Drawing for the job (mm, zero at the part's lowest x, y, z). A direction names the side the tool comes from. Coordinates: 2 decimals unless noted, no trailing zeros. Write each loop counter-clockwise with the first axis right and the second up, starting at its lowest first coordinate (ties: lowest second). Pieces come first, ordered by that corner, then holes. Notation, with made-up numbers: (20, -33) -> (57, -33) arc R28 ccw to (57, -13) -> close; hole circle Ø7 at (22.5, 56). An arc over 180 degrees is marked (long way). Answer as CSV lines item,"result".
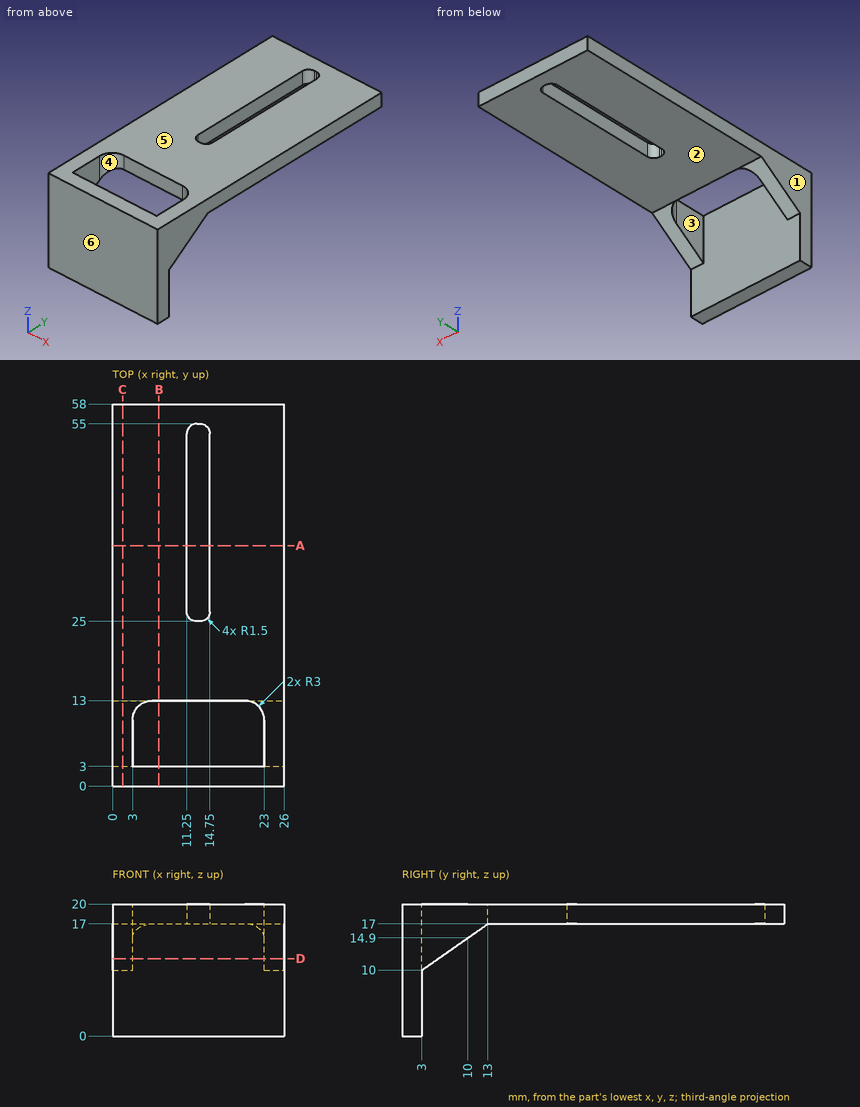
Item 1: 3-axis set-ups, long thin cutter, end or side, ignore diameter. For the marked faces 1, 2 and 3: which of +Z, -Z, +X, -X, +Y, -Y reach the whole face in a straight line?
Answer below:
face 1,"+Z, -Z, -X, +Y, -Y"
face 2,"-Z, +X, -X, +Y"
face 3,"+Z, -Z"
Item 2: Saw through at B-B on x = 7. Give the cut face in (y, z), and give its area (3 significant figures).
Answer below:
outline,"(0, 0) -> (3, 0) -> (3, 20) -> (0, 20) -> close; (13, 17) -> (58, 17) -> (58, 20) -> (13, 20) -> close"
area,"195 mm2"
Item 3: Saw through at C-C on x = 1.5. Give the cut face in (y, z).
Answer below:
outline,"(0, 0) -> (3, 0) -> (3, 10) -> (13, 17) -> (58, 17) -> (58, 20) -> (0, 20) -> close"
Item 4: Wall check: line 1 (Y direction, x = 12.75, z = 18.5); line 2 (X direction, y = 48.5, z = 19.25); line 3 (Y direction, x = 7, z = 18.75). Give the ranges that are in metal, low to high. Write a range as from..to.
Answer below:
line 1,"y = 0..3, 13..25, 55..58"
line 2,"x = 0..11.25, 14.75..26"
line 3,"y = 0..3, 13..58"
Item 5: Saw through at D-D on z = 11.75. Give the cut face in (x, y).
Answer below:
outline,"(0, 0) -> (26, 0) -> (26, 5.5) -> (23, 5.5) -> (23, 3) -> (3, 3) -> (3, 5.5) -> (0, 5.5) -> close"
Item 6: Saw through at A-A on y = 36.5. Give the cut face in (x, z), and give its area (3 significant figures).
Answer below:
outline,"(0, 17) -> (11.25, 17) -> (11.25, 20) -> (0, 20) -> close; (14.75, 17) -> (26, 17) -> (26, 20) -> (14.75, 20) -> close"
area,"67.5 mm2"
Item 7: Two-plate mould, pull along Y, no slides. Class the marked faces 4, 5 and 6: pulls with the +Y half, pulls with the -Y half, needs draft (parallel to the pull), parting line crosses it, or undercut.
Answer below:
face 4,"undercut"
face 5,"needs draft"
face 6,"pulls with the -Y half"
Item 8: Flat gauge pins, fed straight in: pin 1 (2 mm diameter, centred on x = 8.5, z = 4, fed in from +Y); pin 2 (8 mm diameter, centred on x = 6.5, y = 43.5, fed in from -Z); pin 3 (1.5 mm diameter, centred on x = 4, y = 8.5, fed in from +Z). Where does each tip first touch, or does it go through?
Answer below:
pin 1,"stops at y = 3"
pin 2,"stops at z = 17"
pin 3,"passes through"
